from build123d import *

# Parameters (mm, degrees)
F1_DEPTH       = 9.525
F3_D           = 6.35
F3_CBORE_D     = 9.525
F3_CBORE_DEPTH = 3.175
F4_W           = 63.5
F4_H           = 38.1
F8_DEPTH       = 25.4
F10_D          = 12.7
F11_R          = 5.08


with BuildPart() as f1:
    # F0 (on Front) → F1 (new body)
    with BuildSketch(Plane.XZ):
        with BuildLine():
            Line((34.0762832165, 19.05), (-42.1237167835, 19.05))
            ThreePointArc((-42.1237167835, 19.05), (-61.1737167835, 0), (-42.1237167835, -19.05))
            Line((-42.1237167835, -19.05), (34.0762832165, -19.05))
            ThreePointArc((34.0762832165, -19.05), (53.1262832165, 0), (34.0762832165, 19.05))
        make_face()
    extrude(amount=F1_DEPTH)

    # F3 (through all)
    with Locations(Plane.XZ.offset(9.525)):
        with Locations((-48.4737167835, 0), (40.4262832165, 0)):
            CounterBoreHole(F3_D / 2, F3_CBORE_D / 2, F3_CBORE_DEPTH)

    # F6 (on offset) → F7 section 0
    with BuildSketch(Plane.XZ.offset(98.425)):
        with BuildLine():
            Line((16.6010832165, 6.35), (-21.4989167835, 6.35))
            ThreePointArc((-21.4989167835, 6.35), (-27.8489167835, 0), (-21.4989167835, -6.35))
            Line((-21.4989167835, -6.35), (16.6010832165, -6.35))
            ThreePointArc((16.6010832165, -6.35), (22.9510832165, 0), (16.6010832165, 6.35))
        make_face()
    # F4 (on face) → F7 section 1
    with BuildSketch(Plane.XZ.offset(9.525)):
        with Locations((-4.0237167835, 0)):
            Rectangle(F4_W, F4_H)
    loft()

    # F8 (add): a face of the model
    f8_faces = [f1.faces().sort_by_distance(p)[0] for p in [
        (-2.4489167835, -98.425, 0),
    ]]
    extrude(f8_faces, amount=F8_DEPTH)

    # F10 (through all)
    with Locations(Plane(origin=(0, 0, -6.35), x_dir=(1, 0, 0), z_dir=(0, 0, -1))):
        with Locations((-2.4489167835, 111.125)):
            Hole(F10_D / 2)

    # F11
    f11_edges = [f1.edges().sort_by_distance(p)[0] for p in [
        (-27.848917, -123.825, 0),
        (22.951083, -123.825, 0),
        (-2.448917, -123.825, -6.35),
        (-2.448917, -123.825, 6.35),
    ]]
    fillet(f11_edges, radius=F11_R)


solid = f1.part
Could you check a few things on this model? Use its own coordinates, in mm. A direction names the side the tool comes from. Give positions to 0.01 mm unless a question says otherwise; leave off trailing zeros. Order: outer loops, then holes, each group sorted by start corner. A loop starts at its lowest first (then second) coordinate and runs counter-clockwise, first axis right, second up. Notation, with made-up numbers: (6, -25) - (10, -25) arc R12 ccw to (10, -9) - close; hole circle Ø2 at (-16, 71.5). An arc over 180 degrees is marked (long way). Return JSON: item names as keys, results as strings. Group by question number.
Q1. Suppose I cut it at A-A, the plane x = 31.5. Please give me the cut outline in (y, z) (3 decimals).
Q2. Which directions (+Z, -Z, +X, -X, +Y, -Y) give clear straight access to the entire face, cutting with the end or side of a thin tool? Please do faces 1 (the face through (44, -6.35, -1)), 2 (the face through (-3, -104, -6.35)), 3 (the face through (35, -9.525, 0)), 4 (the face through (-43, -9.525, 0)).
Q3. Will these pins go through, and if not, where does the flat tip stop? pin 1 Ø22.5 at (x, y) = (-7.5, -104.5) entering from +Z; pin 2 Ø5 at (x, z) = (-48, 2) entering from -Y; pin 3 Ø12.5 at (x, z) = (-48.47, 0) entering from -Y (3 decimals); pin 4 Ø5.5 at (x, z) = (40.43, 0) entering from +Y.
Q4. Please list where these lines run through material, in increasing order: line 1 along Y through (x, z) = (41.5, 15) (3 decimals); line 2 along Z through (x, y) = (16, -105). Write a range as [from, to].
Q5. Thinking about a two-plate mould opening in Z: for faces 5 (the face through (37.398, -3.131, 0.954)), 6 (the face through (-2.2, -122.4, -4.8)), 7 (the face through (-27.847, -108.443, 0.14)), which applies, pulls with the +Z half, pulls with the -Z half, needs draft (parallel to the pull), parting line crosses it, or undercut?
Resolved:
{
 "1": {"outline": "(-9.525, -19.05) - (0, -19.05) - (0, 19.05) - (-9.525, 19.05) - close"},
 "2": {"face 1": "-Y", "face 2": "-Z, +X, -X, -Y", "face 3": "+Z, -Z, +X, -Y", "face 4": "+Z, -Z, -X, -Y"},
 "3": {"pin 1": "stops at z = 7.09", "pin 2": "stops at y = -6.35", "pin 3": "stops at y = -9.525", "pin 4": "passes through"},
 "4": {"line 1": "y = [-9.525, 0]", "line 2": "z = [-6.35, 6.35]"},
 "5": {"face 5": "undercut", "face 6": "pulls with the -Z half", "face 7": "parting line crosses it"}
}
